Source: CAD feature listing. Evaluate the final solid. Frame: model axes, mm. Face numbers are marked on the shaded views. A direction names the side the tool comes from. Round coordinates to 2 decimals unless told otherwise and drop trailing zeros. Write each loop counter-clockwise with the first axis right and the second up, starting at its lowest first coordinate (ties: lowest second). Pieces come first, ordered by that corner, then holes. Notation, with made-up numbers: (-9.5, -8.75) -> (0.5, -8.75) arc R20 ccw to (0.5, 7.25) -> close; hole circle Ø11 at (22.5, 5). An arc over 180 degrees is marked (long way). Return JSON: item names as keys, results as strings. Group by question number.
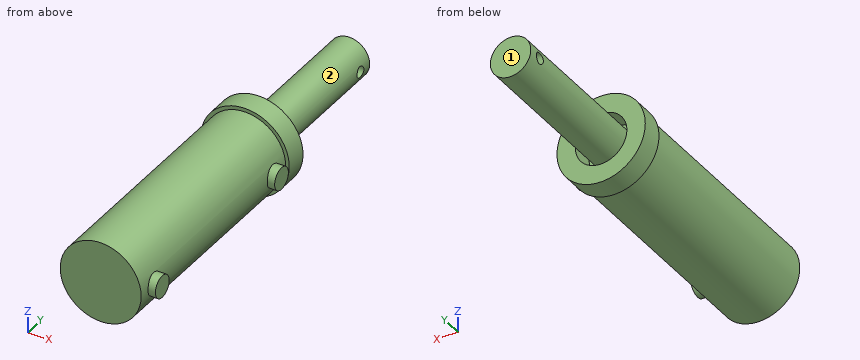
from build123d import *

# Parameters (mm, degrees)
SKETCH1_R               = 69.85
BOSS_EXTRUDE1_DEPTH     = 438.15
SKETCH5_R               = 76.2
BOSS_EXTRUDE5_DEPTH     = 38.1
SKETCH6_R               = 44.45
CUT_EXTRUDE1_DEPTH      = 38.1
BOSS_EXTRUDE7_START     = -12.7
SKETCH8_R               = 19.05
BOSS_EXTRUDE7_DEPTH     = 15.347917
SKETCH9_R               = 34.925
BOSS_EXTRUDE8_DEPTH     = 288.925
SKETCH10_R              = 9.525
CUT_EXTRUDE2_DEPTH      = 83.5500001
CUT_EXTRUDE2_DEPTH_BACK = 77.2


with BuildPart() as part:
    # Sketch1 → Boss-Extrude1 (new body)
    with BuildSketch(Plane(origin=(0, 0, 0), x_dir=(1, 0, 0), z_dir=(0, 1, 0))):
        Circle(SKETCH1_R)
    extrude(amount=BOSS_EXTRUDE1_DEPTH)

    # Sketch5 → Boss-Extrude5 (add)
    with BuildSketch(Plane(origin=(0, 438.15, 0), x_dir=(-1, 0, 0), z_dir=(0, 1, 0))):
        Circle(SKETCH5_R)
    extrude(amount=-BOSS_EXTRUDE5_DEPTH)

    # Sketch6 → Cut-Extrude1 (cut)
    with BuildSketch(Plane(origin=(0, 438.15, 0), x_dir=(1, 0, 0), z_dir=(0, 1, 0))):
        Circle(SKETCH6_R)
    extrude(amount=-CUT_EXTRUDE1_DEPTH, mode=Mode.SUBTRACT)

    # Sketch8 → Boss-Extrude7 (add)
    with BuildSketch(Plane.ZY.offset(-69.85).offset(BOSS_EXTRUDE7_START)):
        with Locations((0, 368.3)):
            Circle(SKETCH8_R)
        with Locations((0, 38.1)):
            Circle(SKETCH8_R)
    extrude(amount=BOSS_EXTRUDE7_DEPTH)

    # Sketch9 → Boss-Extrude8 (add)
    with BuildSketch(Plane(origin=(0, 400.05, 0), x_dir=(1, 0, 0), z_dir=(0, 1, 0))):
        Circle(SKETCH9_R)
    extrude(amount=BOSS_EXTRUDE8_DEPTH)

    # Sketch10 → Cut-Extrude2 (cut, two sides)
    with BuildSketch(Plane(origin=(0, 0, 0), x_dir=(0, 0, -1), z_dir=(1, 0, 0))) as cut_extrude2_sk:
        with Locations((0, 663.575)):
            Circle(SKETCH10_R)
    extrude(amount=CUT_EXTRUDE2_DEPTH, mode=Mode.SUBTRACT)
    extrude(cut_extrude2_sk.sketch, amount=-CUT_EXTRUDE2_DEPTH_BACK, mode=Mode.SUBTRACT)


solid = part.part
Item 1: Cut plane B-B on x = -61. Output: boundary loops of the cut face in (y, z), and give its area (3 significant figures).
Item 2: Set-up query: the marked faces 1 and 2. Return all of +Z, -Z, +X, -X, +Y, -Y with unobstructed straight access to the full face (end or side cutting, diameter ignored); none if empty.
Item 3: Cut plane D-D on z = 52.5. Output: boundary loops of the cut face in (x, y).
Item 4: Cut plane C-C on y = 182.5. Output: boundary loops of the cut face in (x, z).
Item 5: Material intervals for probe 1 along Z at (x, y) = (0, 429) (3 decimals); probe 2 along Y at (x, z) = (-26, 0) (3 decimals); probe 3 along Y at (x, z) = (22, 1) (3 decimals), sorted ascending.
Item 6: First-contact query: pin 1 Ø1 at (x, y) = (-52, 159) entering from +Z; pin 2 Ø6 at (x, y) = (47, 416.5) entering from +Z; pin 3 Ø8 at (x, y) = (-7.5, 521) entering from +Z; pin 4 Ø17 at (y, z) = (663.575, 0) entering from +X. Flat tips, straight axial feed; report the tip coordinate or a pass-through.
Item 7: Cut plane A-A on z = 0. Output: boundary loops of the cut face in (x, y) (3 decimals), and give its area (3 significant figures).
Here are the results:
{
 "1": {"outline": "(0, -34.03) -> (400.05, -34.03) -> (400.05, -45.67) -> (438.15, -45.67) -> (438.15, 45.67) -> (400.05, 45.67) -> (400.05, 34.03) -> (0, 34.03) -> close", "area": "30,700 mm^2"},
 "2": {"face 1": "+Z, -Z, +X, -X, +Y", "face 2": "+Y"},
 "3": {"outline": "(-55.23, 400.05) -> (-46.07, 400.05) -> (-46.07, 0) -> (46.07, 0) -> (46.07, 400.05) -> (55.23, 400.05) -> (55.23, 438.15) -> (-55.23, 438.15) -> close"},
 "4": {"outline": "circle Ø139.7 at (0, 0)"},
 "5": {"probe 1": "z = -76.2 to -44.45, -34.925 to 34.925, 44.45 to 76.2", "probe 2": "y = 0 to 654.05, 673.1 to 688.975", "probe 3": "y = 0 to 654.103, 673.047 to 688.975"},
 "6": {"pin 1": "stops at z = 47.19", "pin 2": "stops at z = 62.21", "pin 3": "stops at z = 34.75", "pin 4": "passes through"},
 "7": {"outline": "(-76.2, 400.05) -> (-69.85, 400.05) -> (-69.85, 0) -> (69.85, 0) -> (69.85, 19.05) -> (82.55, 19.05) -> (82.55, 57.15) -> (69.85, 57.15) -> (69.85, 349.25) -> (82.55, 349.25) -> (82.55, 387.35) -> (69.85, 387.35) -> (69.85, 400.05) -> (76.2, 400.05) -> (76.2, 438.15) -> (44.45, 438.15) -> (44.45, 400.05) -> (34.925, 400.05) -> (34.925, 654.05) -> (-34.925, 654.05) -> (-34.925, 400.05) -> (-44.45, 400.05) -> (-44.45, 438.15) -> (-76.2, 438.15) -> close; (-34.925, 673.1) -> (34.925, 673.1) -> (34.925, 688.975) -> (-34.925, 688.975) -> close", "area": "78,100 mm^2"}
}
